Can you work these out from the model? Positions are in its coordinate system, mm. Face numbers are marked on the shaded views. A direction names the side the tool comes from. Coordinates: 2 decimals unless noted, no trailing zeros. Order: outer loops, then holes, each group sorted by start corner. A loop starts at its lowest first (then second) coordinate and runs counter-clockwise, first axis right, second up. Notation, with made-up numbers: (-35.5, 31) -> (-29.5, 31) arc R31 cw to (-29.5, 56) -> close; hole circle Ø6 at (42.25, -11). An arc over 180 degrees is marked (long way). Use a Markdown table: item, result. Add a question column.
1. For the marked faces 1 and 2, which set-ups out of +Z, -Z, +X, -X, +Y, -Y let a thin tool reach every point of the face, with its end or its side?
2. Suppose I cut it at C-C, the plane z = -132.5. List the corners of the cut face in (x, y) for me, then the cut area to 3 significant figures.
3. If I drill on line 1 along Y through (x, z) = (-0.25, -19); line 2 along Z through (x, y) = (5.75, 1.5); line 3 along Y through (x, z) = (-4.25, -19), over which ranges is the centre line in solid material (lowest first)? Write a range as from..to.
4. For pin 1 Ø8 at (y, z) = (2, -105) entering from +X; pin 2 Ø12 at (x, z) = (7, -90) entering from -Y; pin 3 Ø8 at (x, z) = (6, -86.5) entering from +Y, each with a flat end and sliding along its axis, tell me the tip position at first contact or that it passes through.
5. Suppose I cut it at B-B, the plane z = -19. List the corners of the cut face in (x, y) for me, then the cut area to 3 significant figures.
6. Suppose I cut it at A-A, the plane z = -206. List the corners of the cut face in (x, y) for me, then the cut area to 3 significant figures.
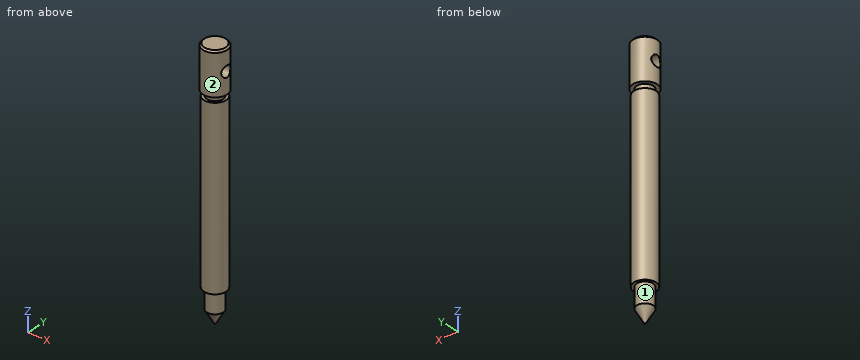
Autodesk Inventor part; units mm, degrees
ref_plane "XZ Plane" through (0, 0, 0) normal (0, 1, 0) x (-1, 0, 0)
ref_plane "XY Plane" through (0, 0, 0) normal (0, 0, 1) x (1, 0, 0)
sketch "Sketch1" plane through (0, 0, 0) normal (1, 0, 0) x (0, 1, 0)
  line L0 (0, 0) -> (9.5, 0)
  line L1 (0, 0) -> (9.5, 0) construction
  line L2 (11, -1.5) -> (11, -38)
  line L3 (11, -38) -> (7.5, -38)
  line L4 (7.5, -38) -> (7.5, -43)
  line L5 (7.5, -43) -> (10, -43)
  line L6 (10, -43) -> (10, -200)
  line L7 (10, -200) -> (7.5, -200)
  line L8 (7.5, -200) -> (7.5, -217.8756)
  line L9 (0.5, -230) -> (0, -230)
  line L10 (0, -230) -> (0, 0)
  line L11 (0.5, -230) -> (7.5, -217.8756)
  line L12 (11, -1.5) -> (9.5, 0)
  line L13 (34.8708, -0.75) -> (56.3474, -0.75)
  line L14 (56.3474, -0.75) -> (56.3474, -28.5061)
  line L15 (56.3474, -28.5061) -> (34.8708, -28.5061)
  line L16 (34.8708, -28.5061) -> (34.8708, -0.75)
  point P0 (11, 0)
  point P1 (7.5, -230)
  point P2 (0.25, -230)
  dimension "d7" = 11
  dimension "d8" = 0
  dimension "d9" = 38
  dimension "d10" = 90
  dimension "d11" = 3.5
  dimension "d12" = 5
  dimension "d13" = 2.5
  dimension "d14" = 157
  dimension "d15" = 90
  dimension "d16" = 2.5
  dimension "d17" = 30
  dimension "d18" = 7.5
  dimension "d19" = 7.25
  dimension "d20" = 7
  dimension "d21" = 60
  dimension "d22" = 1.5
  dimension "d23" = 1.5
revolve "Revolution1" add sketch "Sketch1" angle 360 about axis through (0, 0, -230) along (0, 0, 1) contours L0 L12 L2 L3 L4 L5 L6 L7 L8 L11 L9 L10
thread "Thread1"
sketch "Sketch4" plane through (0, 0, 0) normal (1, 0, 0) x (0, 1, 0)
  circle A0 centre (0, -19) radius 5
  line L0 (9.5, 0) -> (-9.5, 0)
  point P0 (0, 0)
  dimension "d27" = 10
  dimension "d28" = 19
extrude "Extrusion1" cut sketch "Sketch4" along normal mid plane 40
properties part number "atividade_14A_eixo"
Worked out:
| question | item | result |
|---|---|---|
| 1 | face 1 | -Z |
| 1 | face 2 | +Z, -Z |
| 2 | outline | circle Ø20 at (0, 0) |
| 2 | area | 314 mm² |
| 3 | line 1 | y = -11..-5, 5..11 |
| 3 | line 2 | z = -220.57..-23.77, -14.23..0 |
| 3 | line 3 | y = -10.15..-5, 5..10.15 |
| 4 | pin 1 | stops at x = 10 |
| 4 | pin 2 | stops at y = -9.95 |
| 4 | pin 3 | stops at y = 9.8 |
| 5 | outline | (-9.8, -5) arc R11 ccw to (9.8, -5) -> close; (-9.8, 5) -> (9.8, 5) arc R11 ccw to start |
| 5 | area | 168 mm² |
| 6 | outline | circle Ø15 at (0, 0) |
| 6 | area | 177 mm² |
